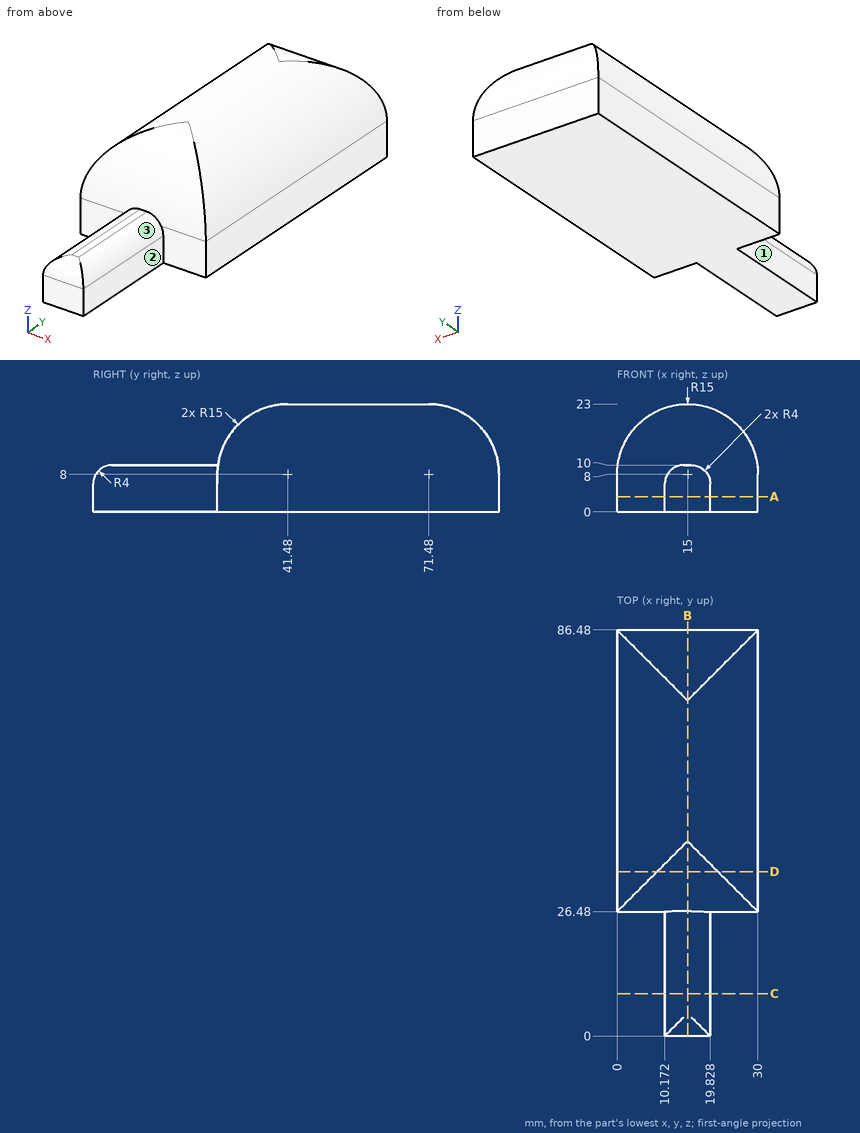
The figure shows three views and two pictorial views of one solid part (mm, origin at its lowest corner). Answer the questions. A direction names the side the tool comes from. Coordinates: 2 decimals unless noted, no trailing zeros. Order: outer loops, then holes, each group sorted by start corner. A loop starts at its lowest first (then second) coordinate and runs counter-clockwise, first axis right, second up.
Q1. Given P1, Ø6.5, axis at x = 25.5, z = 4, coming from the -Y side; P2, Ø6, axis at y = 27.5, z = 20.5, coming from the -X side; P3, Ø3, axis at y = 13, z = 4.5, coming from the +X side; P4, Ø2, axis at x = 7, y = 48, coming from the +Z side, each flat-ended and moving along its own axis, determine where each tip first touches the part or whether it passes through.
Q2. Consider line 1 (Z direction, x = 14.5, y = 5); line 2 (Y direction, x = 8, z = 6.75); line 3 (Z direction, x = 20, y = 67). Determine where each line is inside the solid, lowest interval first.
Q3. A cutting plane is placed at D-D, the plane y = 35. Write down the section's boundary in (x, z).
Q4. Which of the six approach directions +Z, -Z, +X, -X, +Y, -Y give full straight-line access (tool end or side, diameter ignored) to the marked faces 1, 2 and 3?
Q5. A cutting plane is placed at A-A, the plane z = 3.25. Write down the section's boundary in (x, y), and give its area (3 significant figures).
Q6. A cutting plane is placed at C-C, the plane y = 9. Write down the section's boundary in (x, z), and give its area (3 significant figures).
Q7. A cutting plane is placed at B-B, the plane x = 15. Write down the section's boundary in (y, z), and give its area (4 significant figures).
Answers follow:
1. P1: stops at y = 26.48
1. P2: passes through
1. P3: stops at x = 19.83
1. P4: stops at z = 21.27
2. line 1: z = 0 to 10
2. line 2: y = 26.48 to 86.48
2. line 3: z = 0 to 22.14
3. outline: (0, 0) - (30, 0) - (30, 8) arc R15 ccw to (21.48, 21.53) - (8.52, 21.53) arc R15 ccw to (0, 8) - close
4. face 1: +Z, -Z, -X, -Y
4. face 2: +Z, -Z, +X, -Y
4. face 3: +Z, +X, -Y
5. outline: (0, 26.48) - (10.17, 26.48) - (10.17, 0) - (19.83, 0) - (19.83, 26.48) - (30, 26.48) - (30, 86.48) - (0, 86.48) - close
5. area: 2,060 mm2
6. outline: (10.17, 0) - (19.83, 0) - (19.83, 6) arc R4 ccw to (15.83, 10) - (14.17, 10) arc R4 ccw to (10.17, 6) - close
6. area: 89.7 mm2
7. outline: (0, 0) - (86.48, 0) - (86.48, 8) arc R15 ccw to (71.48, 23) - (41.48, 23) arc R15 ccw to (26.61, 10) - (4, 10) arc R4 ccw to (0, 6) - close
7. area: 1,545 mm2
